from build123d import *

# Parameters (mm, degrees)
F1_DEPTH = 50.8
F3_DEPTH = 25.4
F4_W     = 16.1045007408
F4_H     = 10.7811614871
F5_DEPTH = 3.175
F6_W     = 3.2399867196
F6_H     = 27.9691088945
F7_REACH = 85.1871733106
F8_W     = 23.2520068914
F8_H     = 19.5576284379
F9_DEPTH = 3.175
F10_R    = 5.08
F11_R    = 2.54


with BuildPart() as f1:
    # F0 (on Right) → F1 (new body)
    with BuildSketch(Plane.YZ):
        with BuildLine():
            Line((0, 0), (38.4632237256, 0))
            Line((38.4632237256, 0), (38.4632237256, 3.175))
            Line((38.4632237256, 3.175), (18.1845425574, 3.175))
            ThreePointArc((18.1845425574, 3.175), (12.3179075259, 7.0949602045), (13.6944144968, 14.0151280605))
            Line((13.6944144968, 14.0151280605), (54.8708899793, 55.191603543))
            Line((54.8708899793, 55.191603543), (52.2191855315, 57.0300271557))
            Line((52.2191855315, 57.0300271557), (0, 4.8108416242))
            Line((0, 4.8108416242), (0, 0))
        make_face()
    extrude(amount=F1_DEPTH)

    # F2 (on face) → F3 (join)
    with BuildSketch(Plane(origin=(0, -2.4054208121, 2.4054208121), x_dir=(1, 0, 0), z_dir=(0, -0.7071067812, 0.7071067812))):
        Polygon((27.5479931086, 17.2171894163), (50.8, 17.2171894163), (50.8, 36.7748178542), (47.625, 36.7748178542), (47.625, 20.3921894163), (27.5479931086, 20.3921894163), align=None)
    extrude(amount=F3_DEPTH)

    # F4 (on face) → F5 (cut, through all)
    with BuildSketch(Plane(origin=(0, -2.4054208121, 2.4054208121), x_dir=(1, 0, 0), z_dir=(0, -0.7071067812, 0.7071067812))):
        with Locations((8.0522503704, 38.3052378893)):
            Rectangle(F4_W, F4_H)
    extrude(amount=-F5_DEPTH, mode=Mode.SUBTRACT)

    f7_end = Plane(origin=(8.0522503704, 21.9912884712, 24.5570660652), x_dir=(0, 0.7071067812, -0.7071067812), z_dir=(0, 0.7071067812, 0.7071067812))
    # F6 (on Top) → F7 (cut, up to a plane its end follows)
    with BuildSketch(Plane.XY):
        with Locations((1.6199933598, 13.9845544472)):
            Rectangle(F6_W, F6_H)
    f7_long = extrude(amount=F7_REACH, mode=Mode.PRIVATE)
    add(split(f7_long, bisect_by=f7_end, keep=Keep.BOTTOM, mode=Mode.PRIVATE), mode=Mode.SUBTRACT)

    # F8 (on face) → F9 (join)
    with BuildSketch(Plane(origin=(0, -20.3659330543, 20.3659330543), x_dir=(1, 0, 0), z_dir=(0, -0.7071067812, 0.7071067812))):
        with Locations((39.1739965543, 26.9960036352)):
            Rectangle(F8_W, F8_H)
    extrude(amount=F9_DEPTH)

    # F10
    f10_edges = [f1.edges().sort_by_distance(p)[0] for p in [
        (27.019993, 0, 4.810842),
        (50.8, -0.333818, 24.6826),
        (27.547993, 4.515258, 47.492188),
    ]]
    fillet(f10_edges, radius=F10_R)

    # F11
    f11_edges = [f1.edges().sort_by_distance(p)[0] for p in [
        (50.8, 53.545038, 56.110815),
        (50.8, 38.463224, 1.5875),
        (3.239987, 21.991288, 24.557066),
    ]]
    fillet(f11_edges, radius=F11_R)

    # F12: F1 across plane


with BuildPart() as f1_1:
    add(f1.part)
    add(f1.part.mirror(Plane.YZ))


solid = f1_1.part
CAD build for the part. Positions are in the model's coordinates, mm. A direction names the side the tool comes from. Round coordinates to 2 decimals unless told otherwise and drop trailing zeros. Write each loop counter-clockwise with the first axis right and the second up, starting at its lowest first coordinate (ties: lowest second). Pieces come first, ordered by that corner, then holes. Notation, with made-up numbers: M 42,72.5 L 75,72.5 A29 cw 75,102.5 Z; hole C 2,24.5 d3. An arc over 180 degrees is marked long. Use a Markdown table: item, result. Add a question column.
1. Slice it at C-C on y = 26. Give the cut face in (x, z) (1 decimal), then the cut area to 3 significant figures.
2. Slice it at D-D on x = 42. Give the cut face in (y, z) (3 decimals), then the cut area to 4 significant figures.
3. 3-axis set-ups, long thin cutter, end or side, ignore diameter. For faces 1 (the face through (50.036, 37.739, 1.61)), 2 (the face through (36.51, -0.19, 24.54)), 3 (the face through (-37.73, 3.16, 25.68)), 4 (the face through (-27.548, -0.5, 28.9)): which of +Z, -Z, +X, -X, +Y, -Y reach the whole face in a straight line?
4. Drill centre lines: probe 1 along X at (y, z) = (24.5, 26); probe 2 along X at (y, z) = (10.5, 29) (3 decimals); probe 3 along Z at (x, y) = (-9, 16). Where is each one in solid material? Low to high.
5. Slice it at B-B on x = 13. Give the cut face in (y, z) (3 decimals).
6. Slice it at A-A on z = 41. Give the cut face in (x, y) (3 decimals).
7. Pull direction Z, two halves, no side cores. Call faces 5 (the face through (12, 19, 0)), 6 (the face through (3.24, 12, 6)), 7 (the face through (47.625, 9, 32)): released by +Z, released by -Z, zero draft, split by the parting line, or undercut.
8. Flat gauge pins, fed straight in: P1, Ø1, axis at x = 23, z = 1.5, coming from the +Y side; P2, Ø4, axis at x = 13, z = 22.5, coming from the -Y side; P3, Ø6, axis at x = 34.5, y = 47, coming from the -Z side. Where does each tip first touch, or does it go through?
Reply:
| question | item | result |
|---|---|---|
| 1 | outline | M -50.8,0 L -3.2,0 L -3.2,3.2 L -50.8,3.2 Z; M -50.8,26.3 L -16.1,26.3 L -16.1,30.8 L -50.8,30.8 Z; M 3.2,0 L 50.8,0 L 50.8,3.2 L 3.2,3.2 Z; M 16.1,26.3 L 50.8,26.3 L 50.8,30.8 L 16.1,30.8 Z |
| 1 | area | 614 mm^2 |
| 2 | outline | M -10.437,34.785 L 9.769,14.58 L 1.488,6.299 A5.08 ccw 0,2.707 L 0,0 L 38.463,0 L 38.463,3.175 L 18.185,3.175 A6.35 cw 13.694,14.015 L 54.871,55.192 L 52.219,57.03 L 12.014,16.825 L -5.946,34.785 L 5.638,46.37 L 3.393,48.615 Z |
| 2 | area | 550.5 mm^2 |
| 3 | face 1 | -Z, +X, +Y |
| 3 | face 2 | +X, -X, -Y |
| 3 | face 3 | none |
| 3 | face 4 | +Z, -Y |
| 4 | probe 1 | x = -50.8 to -16.1, 16.1 to 50.8 |
| 4 | probe 2 | x = -50.8 to -47.625, 47.625 to 50.8 |
| 4 | probe 3 | z = 0 to 3.56, 16.32 to 20.81 |
| 5 | outline | M 0,0 L 38.463,0 L 38.463,3.175 L 18.185,3.175 A6.35 cw 13.694,14.015 L 23.114,23.435 L 20.869,25.68 L 1.488,6.299 A5.08 ccw 0,2.707 Z; M 28.492,33.303 L 30.737,31.058 L 54.871,55.192 L 52.219,57.03 Z |
| 6 | outline | M -50.8,-4.222 L -27.548,-4.222 L -27.548,0.268 L -47.625,0.268 L -47.625,11.007 L -50.8,11.007 Z; M -50.8,36.189 L 50.8,36.189 L 50.8,40.679 L -50.8,40.679 Z; M 27.548,-4.222 L 50.8,-4.222 L 50.8,11.007 L 47.625,11.007 L 47.625,0.268 L 27.548,0.268 Z |
| 7 | face 5 | released by -Z |
| 7 | face 6 | zero draft |
| 7 | face 7 | undercut |
| 8 | P1 | stops at y = 38.46 |
| 8 | P2 | stops at y = 15.69 |
| 8 | P3 | stops at z = 44.32 |
